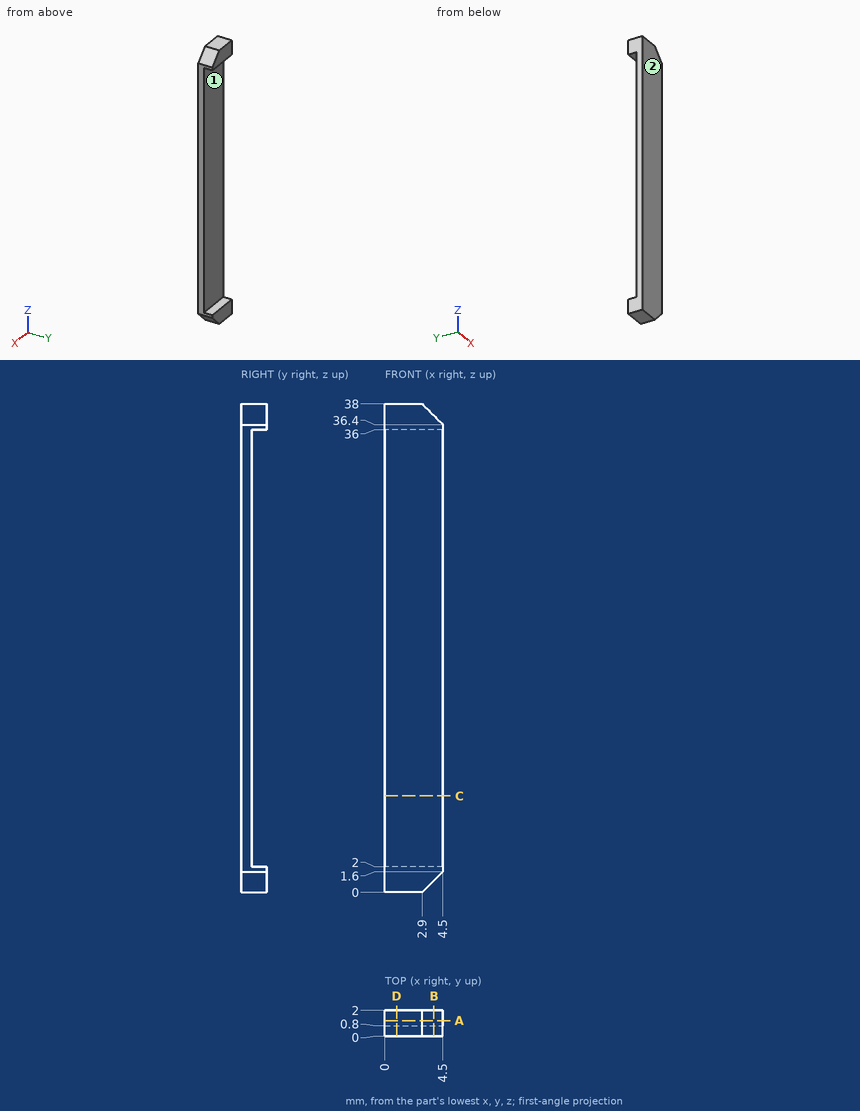
Could you check a few things on this drawing? It's one solid part, dimensions in mm from its lowest x, y, z. Coordinates: 2 decimals unless noted, no trailing zeros. Order: outer loops, then holes, each group sorted by start corner. A loop starts at its lowest first (then second) coordinate and runs counter-clockwise, first axis right, second up.
1. If we section it at D-D (x = 0.9): Please give me the cut outline in (y, z).
2. If we section it at A-A (y = 1.2): Please give me the cut outline in (x, z).
3. If we section it at B-B (x = 3.8): Please give me the cut outline in (y, z), then the cut area to 3 significant figures.
4. If we section it at C-C (z = 7.5): Please give me the cut outline in (x, y), then the cut area to 3 significant figures.
5. I need wall thicknesses on line 1 (Z direction, x = 2.05, y = 1.8); line 2 (Y direction, x = 3.7, z = 6.5); line 3 (Z direction, x = 3.65, y = 1.95). Which ranges of each line are inside material? Lowest first, please.
6. Thinking about a two-plate mould opening in Z: for the marked faces 1 and 2, which applies, +Z half, -Z half, draft (parallel to the pull), parting line (faces both ways), or undercut?
Entries:
1. outline: (0, 0) - (2, 0) - (2, 2) - (0.8, 2) - (0.8, 36) - (2, 36) - (2, 38) - (0, 38) - close
2. outline: (0, 0) - (2.9, 0) - (4.5, 1.6) - (4.5, 2) - (0, 2) - close; (0, 36) - (4.5, 36) - (4.5, 36.4) - (2.9, 38) - (0, 38) - close
3. outline: (0, 0.9) - (2, 0.9) - (2, 2) - (0.8, 2) - (0.8, 36) - (2, 36) - (2, 37.1) - (0, 37.1) - close
3. area: 31.6 mm2
4. outline: (0, 0) - (4.5, 0) - (4.5, 0.8) - (0, 0.8) - close
4. area: 3.60 mm2
5. line 1: z = 0 to 2, 36 to 38
5. line 2: y = 0 to 0.8
5. line 3: z = 0.75 to 2, 36 to 37.25
6. face 1: undercut
6. face 2: draft
